Geometry check sheet. Reference: the model listing, model coordinates, mm. A direction names the side the tool comes from. Give positions to 0.01 mm unless a question says otherwise; leave off trailing zeros. Order: outer loops, then holes, each group sorted by start corner. A loop starts at its lowest first (then second) coordinate and runs counter-clockwise, first axis right, second up. Notation, with made-up numbers: M 88,-13 L 131,-13 A29 cw 131,12 Z; hole C 67,65.5 d2. An arc over 180 degrees is marked long. Answer as a JSON object with one key per item and string values. Group by question number.
from build123d import *

# Parameters (mm, degrees)
BOSS_EXTRUDE1_DEPTH = 4


with BuildPart() as part:
    # Sketch1 → Boss-Extrude1 (new body)
    with BuildSketch(Plane.XY):
        with BuildLine():
            Line((-6.676917421, 3.76), (-6.264383449, 3.76))
            ThreePointArc((-6.264383449, 3.76), (-5.460456542, 3.928688577), (-4.792142921, 4.406298472))
            ThreePointArc((-4.792142921, 4.406298472), (0.997233115, 6.433166103), (5.90126525, 2.748666667))
            ThreePointArc((5.90126525, 2.748666667), (5.414573764, 1.413308514), (4.079215611, 1.9))
            ThreePointArc((4.079215611, 1.9), (0.152344996, 4.497420483), (-3.941291901, 2.171685556))
            ThreePointArc((-3.941291901, 2.171685556), (-4.065842636, 2.023370199), (-4.237411909, 1.933513005))
            ThreePointArc((-4.237411909, 1.933513005), (-4.864598448, 1.796116159), (-5.505, 1.75))
            Line((-5.505, 1.75), (-6.498646087, 1.75))
            ThreePointArc((-6.498646087, 1.75), (-6.995469131, 1.610404776), (-7.492292175, 1.75))
            ThreePointArc((-7.492292175, 1.75), (-10.61, 0), (-7.492292175, -1.75))
            ThreePointArc((-7.492292175, -1.75), (-6.995469131, -1.610404776), (-6.498646087, -1.75))
            Line((-6.498646087, -1.75), (-5.505, -1.75))
            ThreePointArc((-5.505, -1.75), (-4.864598448, -1.796116159), (-4.237411909, -1.933513005))
            ThreePointArc((-4.237411909, -1.933513005), (-4.065842636, -2.023370199), (-3.941291901, -2.171685556))
            ThreePointArc((-3.941291901, -2.171685556), (0.152344996, -4.497420483), (4.079215611, -1.9))
            ThreePointArc((4.079215611, -1.9), (5.414573764, -1.413308514), (5.90126525, -2.748666667))
            ThreePointArc((5.90126525, -2.748666667), (0.997233115, -6.433166103), (-4.792142921, -4.406298472))
            ThreePointArc((-4.792142921, -4.406298472), (-5.460456542, -3.928688577), (-6.264383449, -3.76))
            Line((-6.264383449, -3.76), (-6.676917421, -3.76))
            ThreePointArc((-6.676917421, -3.76), (-6.991575809, -3.784907572), (-7.29839682, -3.859009901))
            ThreePointArc((-7.29839682, -3.859009901), (-12.62, 0), (-7.29839682, 3.859009901))
            ThreePointArc((-7.29839682, 3.859009901), (-6.991575809, 3.784907572), (-6.676917421, 3.76))
        make_face()
    extrude(amount=BOSS_EXTRUDE1_DEPTH)


solid = part.part
1. Cross-section at D-D (y = 0). Record the cut outline in (x, z).
2. Access from +Z, -Z, +X, -X, +Y, -Y to the whole of each face (thin tool, end or side, straight path). Record for faces 4 (the cylindrical face through (-4.874, -1.795, 1.972)), 5 (the cylindrical face through (-5.471, 3.924, 1.972)), 6 (the flat face through (-5, -2, 4)), 7 (the cylindrical face through (-5.45, -3.933, 1.972)).
3. Cross-section at C-C (x = -1). Record the cut outline in (y, z), and give its area (3 significant figures).
4. Thickness scan on line 1 along Y through (x, z) = (-8.56, 1.4); line 2 along X through (y, z) = (0, 1.5); line 3 along Y through (x, z) = (-4, 0.9). Record the ranges inside material, lowest first. Write a range as [from, to].
5. Cross-section at B-B (z = 1.35). Record the cut outline in (x, y) (3 decimals).
6. Depth check by flat-ended pin: pin 1 (1.1 mm diameter, centred on x = -6, z = 3, fed in from -Y); pin 2 (0.5 mm diameter, centred on x = -6.5, z = 3, fed in from -Y); pin 3 (0.5 mm diameter, centred on x = -6, z = 1.5, fed in from +Y). Enter the tip coordinate at first touch or a pass-through.
7. Cross-section at A-A (x = -8.56). Record the cut outline in (y, z), and give its area (3 significant figures).
8. Release check for a two-part mould opening along X. For faces 1 (the flat face through (-5, -2, 0)), 2 (the cylindrical face through (5.43, 1.42, 1.97)), 3 (the cylindrical face through (0.909, 6.446, 1.972)) record: released by +X, released by -X, zero draft, split by the parting line, or undercut.
Report:
{
 "1": {"outline": "M -12.62,0 L -10.61,0 L -10.61,4 L -12.62,4 Z"},
 "2": {"face 4": "+Z, -Z", "face 5": "+Z, -Z, +Y", "face 6": "+Z, +X, -X, +Y, -Y", "face 7": "+Z, -Z, -Y"},
 "3": {"outline": "M -6.43,0 L -4.39,0 L -4.39,4 L -6.43,4 Z; M 4.39,0 L 6.43,0 L 6.43,4 L 4.39,4 Z", "area": "16.4 mm2"},
 "4": {"line 1": "y = [-4.06, -2.05], [2.05, 4.06]", "line 2": "x = [-12.62, -10.61]", "line 3": "y = [-5.14, -2.09], [2.09, 5.14]"},
 "5": {"outline": "M -7.492,-1.75 A2.05 cw long -7.492,1.75 A0.954 ccw -6.499,1.75 L -5.505,1.75 A4.47 ccw -4.237,1.934 A0.5 ccw -3.941,2.172 A4.5 cw 4.079,1.9 A1.005 ccw 5.901,2.749 A6.51 ccw -4.792,4.406 A2 cw -6.264,3.76 L -6.677,3.76 A2 cw -7.298,3.859 A4.06 ccw long -7.298,-3.859 A2 cw -6.677,-3.76 L -6.264,-3.76 A2 cw -4.792,-4.406 A6.51 ccw 5.901,-2.749 A1.005 ccw 4.079,-1.9 A4.5 cw -3.941,-2.172 A0.5 ccw -4.237,-1.934 A4.47 ccw -5.505,-1.75 L -6.499,-1.75 A0.954 ccw Z"},
 "6": {"pin 1": "stops at y = -3.93", "pin 2": "stops at y = -3.76", "pin 3": "stops at y = 3.83"},
 "7": {"outline": "M -4.06,0 L -2.05,0 L -2.05,4 L -4.06,4 Z; M 2.05,0 L 4.06,0 L 4.06,4 L 2.05,4 Z", "area": "16.1 mm2"},
 "8": {"face 1": "zero draft", "face 2": "undercut", "face 3": "split by the parting line"}
}
